from build123d import *

# Parameters (mm, degrees)
SKETCH1_W           = 10
SKETCH1_H           = 10
SKETCH1_W_2         = 7
SKETCH1_H_2         = 7
BOSS_EXTRUDE1_DEPTH = 3
SKETCH2_W           = 10
SKETCH2_H           = 10
BOSS_EXTRUDE2_DEPTH = 1
SKETCH3_R           = 2.5
BOSS_EXTRUDE3_DEPTH = 12.5
FILLET1_R           = 1


with BuildPart() as part:
    # Sketch1 → Boss-Extrude1 (new body)
    with BuildSketch(Plane(origin=(0, 0, 0), x_dir=(1, 0, 0), z_dir=(0, 1, 0))):
        with Locations((5, 5)):
            Rectangle(SKETCH1_W, SKETCH1_H)
        with Locations((5, 5)):
            Rectangle(SKETCH1_W_2, SKETCH1_H_2, mode=Mode.SUBTRACT)
    extrude(amount=BOSS_EXTRUDE1_DEPTH)

    # Sketch2 → Boss-Extrude2 (add)
    with BuildSketch(Plane(origin=(0, 3, 0), x_dir=(1, 0, 0), z_dir=(0, 1, 0))):
        with Locations((5, 5)):
            Rectangle(SKETCH2_W, SKETCH2_H)
    extrude(amount=BOSS_EXTRUDE2_DEPTH)

    # Sketch3 → Boss-Extrude3 (add)
    with BuildSketch(Plane(origin=(0, 4, 0), x_dir=(1, 0, 0), z_dir=(0, 1, 0))):
        with Locations((5, 5)):
            Circle(SKETCH3_R)
    extrude(amount=BOSS_EXTRUDE3_DEPTH)

    # Fillet1
    fillet1_edges = [part.edges().sort_by_distance(p)[0] for p in [
        (2.5, 16.5, -5),
        (0, 2, -10),
        (10, 2, -10),
        (10, 2, 0),
        (0, 2, 0),
    ]]
    fillet(fillet1_edges, radius=FILLET1_R)


solid = part.part
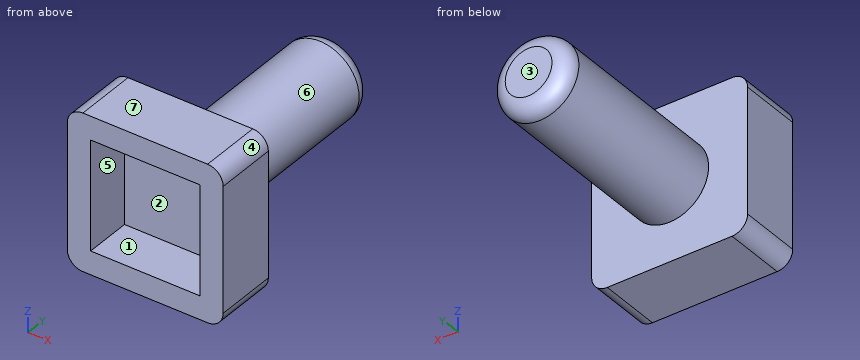
Source: CAD feature listing. Evaluate the final solid. Frame: model axes, mm. Face numbers are marked on the shaded views. A direction names the side the tool comes from. Round coordinates to 2 decimals unless told otherwise and drop trailing zeros. Loops run counter-clockwise (first coordinate to the right, second up) from the corner with the lowest first, then second, coordinate; pieces in that order, holes last. Notation, with made-up numbers: (-9, -8) - (39, -8) arc R22 ccw to (39, 3) - close; hole circle Ø2 at (-22, 54). An arc over 180 degrees is marked (long way). Write item = value, one per line. Start each with the question number.
Item 1: Section query B-B on y = 2.75. Output: boundary loops of the cut face in (x, z).
Item 2: Section query A-A on x = 1.75. Output: boundary loops of the cut face in (y, z).
Item 3: Reachability of the marked faces 5, 6 and 7 from +Z, -Z, +X, -X, +Y, -Y: full face, straight path, thin tool, end or side. Return the list, or none.
Item 4: First-contact query: pin 1 Ø1.5 at (x, z) = (2, -7) entering from -Y; pin 2 Ø6 at (y, z) = (10.5, -4.5) entering from -X; pin 3 Ø2 at (x, z) = (6, -5) entering from -Y; pin 4 Ø6 at (x, y) = (7.5, 10.5) entering from -Z. Flat tips, straight axial feed; report the tip coordinate or a pass-through.
Item 5: Section query C-C on z = -5. Output: boundary loops of the cut face in (x, y).
Item 6: Section query D-D on y = 8. Output: boundary loops of the cut face in (x, z).
Item 7: Material intervals for line 1 (X direction, y = 2.5, z = -2); line 2 (X direction, y = 14.75, z = -3); line 3 (Y direction, x = 7.5, z = -1.25), sorted ascending.
Item 8: Mould query, pull axis Z, two halves, no side actions, for the marked faces 1, 2, 3 and 4. Classes: released by +Z, released by -Z, zero draft, split by the parting line, or undercut.
Results list:
q1.outline = (0, -9) arc R1 ccw to (1, -10) - (9, -10) arc R1 ccw to (10, -9) - (10, -1) arc R1 ccw to (9, 0) - (1, 0) arc R1 ccw to (0, -1) - close; hole (1.5, -8.5) - (8.5, -8.5) - (8.5, -1.5) - (1.5, -1.5) - close
q2.outline = (0, -10) - (4, -10) - (4, 0) - (0, 0) - (0, -1.5) - (3, -1.5) - (3, -8.5) - (0, -8.5) - close
q3.face_5 = -Y
q3.face_6 = +Y
q3.face_7 = +Z, +X, -X, +Y, -Y
q4.pin_1 = 0
q4.pin_2 = 2.5
q4.pin_3 = 3
q4.pin_4 = -7.5
q5.outline = (0, 0) - (1.5, 0) - (1.5, 3) - (8.5, 3) - (8.5, 0) - (10, 0) - (10, 4) - (7.5, 4) - (7.5, 15.5) arc R1 ccw to (6.5, 16.5) - (3.5, 16.5) arc R1 ccw to (2.5, 15.5) - (2.5, 4) - (0, 4) - close
q6.outline = circle Ø5 at (5, -5)
q7.line_1 = 0 to 1.5, 8.5 to 10
q7.line_2 = 3.5 to 6.5
q7.line_3 = 0 to 4
q8.face_1 = undercut
q8.face_2 = undercut
q8.face_3 = zero draft
q8.face_4 = released by +Z
